from build123d import *

# Parameters (mm, degrees)
F1_DEPTH  = 150
F2_DEPTH  = 147
F3_W      = 51
F3_H      = 91
F3_W_2    = 45
F3_H_2    = 85
F4_DEPTH  = 17
F5_DEPTH  = 15
F6_W      = 85
F6_H      = 9
F7_DEPTH  = 75
F8_W      = 45.0000017881
F8_H      = 9.0000017881
F9_DEPTH  = 95
F10_W     = 2.6170494705
F10_H     = 25
F11_DEPTH = 25


with BuildPart() as f1:
    # F0 (on Front) → F1 (new body)
    with BuildSketch(Plane.XZ):
        Polygon((-44.3471273035, 8.3293294263), (-29.3471273035, 8.3293294263), (-29.3471273035, 10.3293294263), (-30.6854649693, 10.3293294263), (-32.7072627842, 10.3293294263), (-44.3471273035, 10.3293294263), align=None)
        Polygon((-29.3471273035, -10.1195359603), (29.6528726965, -10.1195359603), (29.6528726965, 8.3293294263), (29.6528726965, 10.3293294263), (29.6528726965, 14.3293294263), (27.6528726965, 14.3293294263), (27.6528726965, 10.3293294263), (27.6528726965, 9.2171130797), (27.6528726965, -8.1195359603), (-27.3471273035, -8.1195359603), (-27.3471273035, 9.2171130797), (-27.3471273035, 10.3293294263), (-27.3471273035, 14.3293294263), (-29.3471273035, 14.3293294263), (-29.3471273035, 10.3293294263), (-29.3471273035, 8.3293294263), align=None)
        Polygon((29.6528726965, 10.3293294263), (29.6528726965, 8.3293294263), (44.6528726965, 8.3293294263), (44.6528726965, 10.3293294263), (41.5029401332, 10.3293294263), (33.3236008883, 10.3293294263), align=None)
    extrude(amount=-F1_DEPTH)

    # F0 (on Front) → F2 (join)
    with BuildSketch(Plane.XZ):
        with BuildLine():
            Line((29.6528726965, 14.3293294263), (29.6528726965, 10.3293294263))
            Line((29.6528726965, 10.3293294263), (33.3236008883, 10.3293294263))
            ThreePointArc((33.3236008883, 10.3293294263), (30.709634425, 11.6148200112), (29.6528726965, 14.3293294263))
        make_face()
        with BuildLine():
            Line((-30.6854649693, 10.3293294263), (-29.3471273035, 10.3293294263))
            Line((-29.3471273035, 10.3293294263), (-29.3471273035, 14.3293294263))
            ThreePointArc((-29.3471273035, 14.3293294263), (-30.2986339381, 11.7173134209), (-32.7072627842, 10.3293294263))
            Line((-32.7072627842, 10.3293294263), (-30.6854649693, 10.3293294263))
        make_face()
    extrude(amount=-F2_DEPTH)

    # F3 (on face) → F4 (join)
    with BuildSketch(Plane.XY.offset(-8.1195359603)):
        with Locations((0, 75.1699954271)):
            Rectangle(F3_W, F3_H)
        with Locations((0, 75.1699954271)):
            Rectangle(F3_W_2, F3_H_2, mode=Mode.SUBTRACT)
        with Locations((0, 75.1699954271)):
            Rectangle(F3_W_2, F3_H_2)
    extrude(amount=-F4_DEPTH)

    # F3 (on face) → F5 (cut)
    with BuildSketch(Plane.XY.offset(-8.1195359603)):
        with Locations((0, 75.1699954271)):
            Rectangle(F3_W_2, F3_H_2)
    extrude(amount=-F5_DEPTH, mode=Mode.SUBTRACT)

    # F6 (on face) → F7 (cut)
    with BuildSketch(Plane.YZ.offset(25.5)):
        with Locations((75.1699954271, -17.6195359603)):
            Rectangle(F6_W, F6_H)
    extrude(amount=-F7_DEPTH, mode=Mode.SUBTRACT)

    # F8 (on face) → F9 (cut)
    with BuildSketch(Plane.XZ.offset(-29.6699954271)):
        with Locations((0, -17.6195359603)):
            Rectangle(F8_W, F8_H)
    extrude(amount=-F9_DEPTH, mode=Mode.SUBTRACT)

    # F10 (on face) → F11 (cut)
    with BuildSketch(Plane(origin=(0, 0, 8.3293294263), x_dir=(1, 0, 0), z_dir=(0, 0, -1))):
        Polygon((-29.5194201171, -23.8912090659), (-29.7296848148, -23.8912090659), (-32.3471273035, -23.8912090659), (-32.3471273035, -48.8912090659), (-29.7296848148, -48.8912090659), (-29.5194201171, -48.8912090659), (-29.5194201171, -48.8749593496), align=None)
        with Locations((31.0386025682, -36.3912090659)):
            Rectangle(F10_W, F10_H)
        with Locations((31.0386025682, -113.6087909341)):
            Rectangle(F10_W, F10_H)
        Polygon((-29.5194201171, -101.1250406504), (-29.5194201171, -101.1087909341), (-29.7296848148, -101.1087909341), (-32.3471273035, -101.1087909341), (-32.3471273035, -126.1087909341), (-29.7296848148, -126.1087909341), (-29.5194201171, -126.1087909341), align=None)
    extrude(amount=-F11_DEPTH, mode=Mode.SUBTRACT)


solid = f1.part
Model file for the job. Use its own axes, mm. A direction names the side the tool comes from. Give positions to 0.01 mm unless a question says otherwise; leave off trailing zeros. Loops run counter-clockwise (first coordinate to the right, second up) from the corner with the lowest first, then second, coordinate; pieces in that order, holes last. Notation, with made-up numbers: (73.5, 3) -> (99.5, 3) arc R20 ccw to (99.5, 12) -> close; hole circle Ø7 at (19.5, 47.25). An arc over 180 degrees is marked (long way). Use a Markdown table: item, result. Add a question column.
(1) Wall check: line 1 along X through (y, z) = (115, 8.5); line 2 along X through (y, z) = (10.5, 2.5); line 3 along Y through (x, z) = (5, -11.5). Give the ranges that are in metal, low to high.
(2) Slice it at B-B on x = 11.5. List the corners of the cut face in (y, z).
(3) Slice it at D-D on y = 96. Give the number of separate pieces and of enclosed holes in the cut face, and give its area (3 significant figures).
(4) Mould opens along Z. For faces 1 (the flat face through (27.653, 74, 3)), 2 (the flat face through (22.5, 31, -18)), 3 (the flat face through (-24, 75, -13.12)), 4 (the cylindrical face through (30.74, 72.47, 11.58)) say: +Z half, -Z half, draft (parallel to the pull), parting line (faces both ways), or undercut.
(5) Slice it at A-A on z = -17. List the corners of the cut face in (x, y).
(6) Tool access for faces 5 (the flat face through (25.5, 75, -23)), 6 (the flat face through (-22.5, 31, -18)), 7 (the flat face through (-37, 74, 8.329)): list every direction of +Z, -Z, +X, -X, +Y, -Y with a clear straight run to the whole face (end or side of a thin tool).
(7) Drop flat-ended pins along their axis: pin 1 Ø0.9 at (x, y) = (24.5, 74) entering from +Z; pin 2 Ø7.5 at (x, y) = (34, 52.5) entering from +Z; pin 3 Ø10 at (x, z) = (-9, -3.5) entering from +Y; pin 4 Ø2.5 at (x, z) = (0, -11.5) entering from -Y. Give the stop position or say it passes through.
(8) Slice it at C-C on z = 4. List the corners of the cut face in (x, y).
Filled sheet:
| question | item | result |
|---|---|---|
| 1 | line 1 | -44.35 to -32.35, -29.52 to -27.35, 27.65 to 29.73, 32.35 to 44.65 |
| 1 | line 2 | -29.35 to -27.35, 27.65 to 29.65 |
| 1 | line 3 | 29.67 to 32.67, 117.67 to 120.67 |
| 2 | outline | (0, -10.12) -> (29.67, -10.12) -> (29.67, -13.12) -> (32.67, -13.12) -> (32.67, -8.12) -> (0, -8.12) -> close; (29.67, -25.12) -> (120.67, -25.12) -> (120.67, -22.12) -> (117.67, -22.12) -> (117.67, -23.12) -> (32.67, -23.12) -> (32.67, -22.12) -> (29.67, -22.12) -> close; (117.67, -13.12) -> (120.67, -13.12) -> (120.67, -10.12) -> (150, -10.12) -> (150, -8.12) -> (117.67, -8.12) -> close |
| 3 | separate pieces | 3 |
| 3 | enclosed holes | 0 |
| 3 | area | 311 mm2 |
| 4 | face 1 | draft |
| 4 | face 2 | undercut |
| 4 | face 3 | undercut |
| 4 | face 4 | +Z half |
| 5 | outline | (-25.5, 29.67) -> (-22.5, 29.67) -> (-22.5, 32.67) -> (-25.5, 32.67) -> close; (-25.5, 117.67) -> (-22.5, 117.67) -> (-22.5, 120.67) -> (-25.5, 120.67) -> close; (22.5, 29.67) -> (25.5, 29.67) -> (25.5, 32.67) -> (22.5, 32.67) -> close; (22.5, 117.67) -> (25.5, 117.67) -> (25.5, 120.67) -> (22.5, 120.67) -> close |
| 6 | face 5 | -Z, +X, +Y, -Y |
| 6 | face 6 | +Y, -Y |
| 6 | face 7 | -Z, -X, +Y, -Y |
| 7 | pin 1 | z = -8.12 |
| 7 | pin 2 | z = 12.22 |
| 7 | pin 3 | y = 150 |
| 7 | pin 4 | y = 29.67 |
| 8 | outline | (-29.35, 0) -> (-27.35, 0) -> (-27.35, 150) -> (-29.35, 150) -> close; (27.65, 0) -> (29.65, 0) -> (29.65, 150) -> (27.65, 150) -> close |
